from build123d import *
from build123d.topology import SkipClean

# Parameters (mm, degrees)
SKETCH_1_R          = 11
SKETCH_1_R_2        = 5
SKETCH_1_R_3        = 1.1
EXTRUDE_1_DEPTH     = 3
EXTRUDE_2_DEPTH     = 5.5
EXTRUDE_3_DEPTH     = 7.1
CHAMFER_1_SIZE      = 3
CUT_EXTRUDE_1_DEPTH = 10
CUT_EXTRUDE_2_REACH = 19.1
SKETCH_5_R          = 1.1


with BuildPart() as part:
    # 草图1 → 凸台-拉伸1 (new body)
    with BuildSketch(Plane.XY):
        Circle(SKETCH_1_R)
        Circle(SKETCH_1_R_2, mode=Mode.SUBTRACT)
        with Locations((-6.5, 0)):
            Circle(SKETCH_1_R_3, mode=Mode.SUBTRACT)
        with Locations((6.5, 0)):
            Circle(SKETCH_1_R_3, mode=Mode.SUBTRACT)
    extrude(amount=EXTRUDE_1_DEPTH)

    # 草图2 → 凸台-拉伸2 (add)
    with SkipClean():  # the faces are left unmerged after this step: merging them gives an invalid solid
        with BuildSketch(Plane.XY.offset(3)):
            with BuildLine():
                ThreePointArc((4.865384615, -1.152402944), (8.5, 0), (4.865384615, 1.152402944))
                ThreePointArc((4.865384615, 1.152402944), (5, 0), (4.865384615, -1.152402944))
            make_face()
            with BuildLine():
                ThreePointArc((-4.865384615, 1.152402944), (-8.5, 0), (-4.865384615, -1.152402944))
                ThreePointArc((-4.865384615, -1.152402944), (-5, 0), (-4.865384615, 1.152402944))
            make_face()
        extrude(amount=EXTRUDE_2_DEPTH)

    # 草图3 → 凸台-拉伸3 (add)
    with SkipClean():  # the faces are left unmerged after this step: merging them gives an invalid solid
        with BuildSketch(Plane.XY.offset(3)):
            with BuildLine():
                Line((-6.60837923, -8.79370934), (-6, -7.984144705))
                ThreePointArc((-6, -7.984144705), (0, 9.987320295), (6, -7.984144705))
                Line((6, -7.984144705), (6.60837923, -8.79370934))
                ThreePointArc((6.60837923, -8.79370934), (0, 11), (-6.60837923, -8.79370934))
            make_face()
        extrude(amount=EXTRUDE_3_DEPTH)

    # 倒角1
    # the kernel refuses this chamfer: 3 mm, written as the material it adds along each edge
    with BuildSketch(Plane(origin=(6.5, 0, 3), x_dir=(-0.9999950652018583, -0.0031415874858795587, 0), z_dir=(-0.0031415874858795587, 0.9999950652018583, 0))) as chamfer_1_piece_1_section:
        Polygon((2 + CHAMFER_1_SIZE, 0), (2, CHAMFER_1_SIZE), (2, 0), align=None)
    chamfer_1_piece_1 = revolve(axis=Axis((6.5, 0, 3), (0, 0, 1)), revolution_arc=359.64, mode=Mode.PRIVATE)
    chamfer_1_piece_1 = chamfer_1_piece_1 - Plane(origin=(0, 0, 3.47273438), x_dir=(1, 0, 0), z_dir=(0, 0, -1)) * Cylinder(5, 21, mode=Mode.PRIVATE)
    chamfer_1_piece_1 = chamfer_1_piece_1 & Plane(origin=(0, 0, 3.47273438), x_dir=(-0.6007617481958082, -0.7994281217875167, 0), z_dir=(0, 0, -1)) * Cylinder(9.987320295, 21, mode=Mode.PRIVATE)
    add(chamfer_1_piece_1)
    with BuildSketch(Plane(origin=(-6.5, 0, 3), x_dir=(0.9999950652018583, 0.0031415874858795045, 0), z_dir=(0.0031415874858795045, -0.9999950652018583, 0))) as chamfer_1_piece_2_section:
        Polygon((2 + CHAMFER_1_SIZE, 0), (2, CHAMFER_1_SIZE), (2, 0), align=None)
    chamfer_1_piece_2 = revolve(axis=Axis((-6.5, 0, 3), (0, 0, 1)), revolution_arc=359.64, mode=Mode.PRIVATE)
    chamfer_1_piece_2 = chamfer_1_piece_2 - Plane(origin=(0, 0, 3.472734386), x_dir=(1, 0, 0), z_dir=(0, 0, -1)) * Cylinder(5, 21, mode=Mode.PRIVATE)
    chamfer_1_piece_2 = chamfer_1_piece_2 & Plane(origin=(0, 0, 3.472734386), x_dir=(-0.6007617481958082, -0.7994281217875167, 0), z_dir=(0, 0, -1)) * Cylinder(9.987320295, 21, mode=Mode.PRIVATE)
    add(chamfer_1_piece_2)

    # 草图4 → 切除-拉伸1 (cut)
    with BuildSketch(Plane(origin=(0, 0, 0), x_dir=(-1, 0, 0), z_dir=(0, 0, -1))):
        with BuildLine():
            ThreePointArc((-6.60837923, -8.79370934), (0, -11), (6.60837923, -8.79370934))
            Line((6.60837923, -8.79370934), (3.003808741, -3.997140609))
            ThreePointArc((3.003808741, -3.997140609), (0, -5), (-3.003808741, -3.997140609))
            Line((-3.003808741, -3.997140609), (-6.60837923, -8.79370934))
        make_face()
    extrude(amount=-CUT_EXTRUDE_1_DEPTH, mode=Mode.SUBTRACT)

    # 草图5 → 切除-拉伸2 (cut, up to next)
    with BuildSketch(Plane(origin=(0, 0, 3), x_dir=(-1, 0, 0), z_dir=(0, 0, -1)), mode=Mode.PRIVATE) as cut_extrude_2_sk1:
        with Locations(Location((6.5, 0, 0), (0, 0, 180))):
            Circle(SKETCH_5_R)
    cut_extrude_2_tool1 = extrude(cut_extrude_2_sk1.sketch, amount=-CUT_EXTRUDE_2_REACH, mode=Mode.PRIVATE) & part.part
    # 草图5 → 切除-拉伸2 (cut, up to next)
    with BuildSketch(Plane(origin=(0, 0, 3), x_dir=(-1, 0, 0), z_dir=(0, 0, -1)), mode=Mode.PRIVATE) as cut_extrude_2_sk2:
        with Locations(Location((-6.5, 0, 0), (0, 0, 180))):
            Circle(SKETCH_5_R)
    cut_extrude_2_tool2 = extrude(cut_extrude_2_sk2.sketch, amount=-CUT_EXTRUDE_2_REACH, mode=Mode.PRIVATE) & part.part
    add(cut_extrude_2_tool1.solids().sort_by_distance((-6.5, 0, 3))[0], mode=Mode.SUBTRACT)
    add(cut_extrude_2_tool2.solids().sort_by_distance((6.5, 0, 3))[0], mode=Mode.SUBTRACT)


solid = part.part
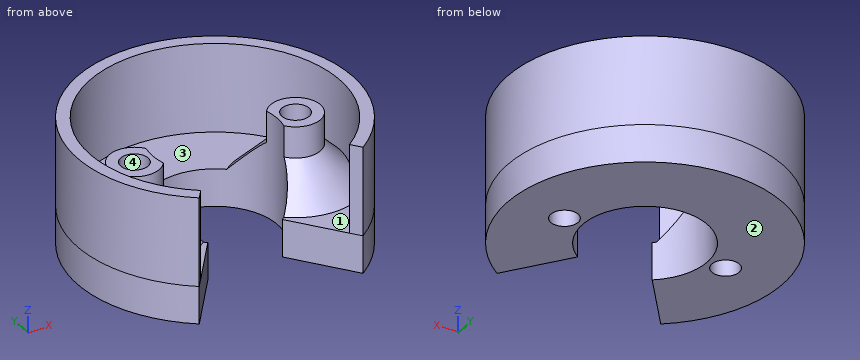
The model under review builds one solid part; all positions refer to its coordinate system, in mm. Face numbers are marked on the shaded views. A direction names the side the tool comes from. Round coordinates to 2 decimals unless told otherwise and drop trailing zeros. Loops run counter-clockwise (first coordinate to the right, second up) from the corner with the lowest first, then second, coordinate; pieces in that order, holes last. Notation, with made-up numbers: (-31, -12) -> (3, -12) arc R24 cw to (3, 4) -> close; hole circle Ø11 at (-35, 30.25). An arc over 180 degrees is marked (long way). One line per question, with ' | ' between items. Start each with the question number.
Item 1: Add section A-A, the plane z = 6.5. Write out the cut boundary in (x, y), then the cut area to 3 significant figures.
Item 2: Machinability: for the marked faces 3 and 4, which of the approach directions +Z, -Z, +X, -X, +Y, -Y give a long, thin tool a straight path to every point of the face, cutting with its end or side? Answer none if there is none.
Item 3: Wall thickness on line 1 along X through (y, z) = (0, 2); line 2 along X through (y, z) = (0, 5.75); line 3 along Y through (x, z) = (-6.75, 4.5): over which ranges is each line inside the solid? List them lowest first. Write a range as [from, to].
Item 4: For pin 1 (1.5 mm diameter, centred on x = 7.5, y = 0.5, fed in from -Z); pin 2 (4 mm diameter, centred on x = 7.5, y = 0, fed in from +Z); pin 3 (1.9 mm diameter, centred on x = 2, y = 7.5, fed in from +Z); pin 4 (3 mm diameter, centred on y = -6.5, z = 1.5, fed in from -X), all flat-tipped, find the tip position at first contact; note any pin that passes through.
Item 5: Add section D-D, the plane y = 0. Write out the cut boundary in (x, z).
Item 6: Draft analysis for pull direction Y (two halves, no side actions). For the marked faces 1 and 2, state which applies: +Y half, -Y half, draft (parallel to the pull), parting line (faces both ways), or undercut.
Item 7: Add section B-B, the plane y = -5.75. Write out the cut boundary in (x, z), then the cut area to 3 significant figures.
Item 8: Add section C-C, the plane z = 1.25. Write out the cut boundary in (x, y), then the cut area to 3 significant figures.
Return value:
1) outline: (-6.61, -8.79) -> (-6, -7.98) arc R9.99 cw (long way) to (6, -7.98) -> (6.61, -8.79) arc R11 ccw (long way) to start; (-4.87, -1.15) arc R5 cw to (-4.87, 1.15) arc R2 ccw (long way) to start; (4.87, -1.15) arc R2 ccw (long way) to (4.87, 1.15) arc R5 cw to start; hole circle Ø2.2 at (-6.5, 0); hole circle Ø2.2 at (6.5, 0) | area: 69.0 mm2
2) face 3: +Z | face 4: +Z, -Z
3) line 1: x = [-11, -7.6], [-5.4, -5], [5, 5.4], [7.6, 11] | line 2: x = [-11, -9.99], [-8.75, -7.6], [-5.4, -5], [5, 5.4], [7.6, 8.75], [9.99, 11] | line 3: y = [-8.69, -7.36], [-3.49, -1.07], [1.07, 3.49], [7.36, 8.69]
4) pin 1: stops at z = 0 | pin 2: stops at z = 8.5 | pin 3: stops at z = 3 | pin 4: stops at x = -9.8
5) outline: (-11, 0) -> (-7.6, 0) -> (-7.6, 8.5) -> (-8.5, 8.5) -> (-8.5, 6) -> (-9.99, 4.51) -> (-9.99, 10.1) -> (-11, 10.1) -> close; (-5.4, 0) -> (-5, 0) -> (-5, 8.5) -> (-5.4, 8.5) -> close; (5, 0) -> (5.4, 0) -> (5.4, 8.5) -> (5, 8.5) -> close; (7.6, 0) -> (11, 0) -> (11, 10.1) -> (9.99, 10.1) -> (9.99, 4.51) -> (8.5, 6) -> (8.5, 8.5) -> (7.6, 8.5) -> close
6) face 1: undercut | face 2: draft
7) outline: (-9.38, 0) -> (-4.32, 0) -> (-4.32, 3) -> (-8.17, 3) -> (-8.17, 10.1) -> (-9.38, 10.1) -> close; (4.32, 0) -> (9.38, 0) -> (9.38, 10.1) -> (8.17, 10.1) -> (8.17, 3) -> (4.32, 3) -> close | area: 47.5 mm2
8) outline: (-6.61, -8.79) -> (-3, -4) arc R5 cw (long way) to (3, -4) -> (6.61, -8.79) arc R11 ccw (long way) to start; hole circle Ø2.2 at (-6.5, 0); hole circle Ø2.2 at (6.5, 0) | area: 232 mm2
